Here's the drawing with two shaded views (mm, measured from the low corner). I have some questions. A direction names the side the tool comes from. Give positions to 0.01 mm unless a question says otherwise; leave off trailing zeros. Write each loop counter-clockwise with the first axis right and the second up, starting at its lowest first coordinate (ties: lowest second). Pieces come first, ordered by that corner, then holes.
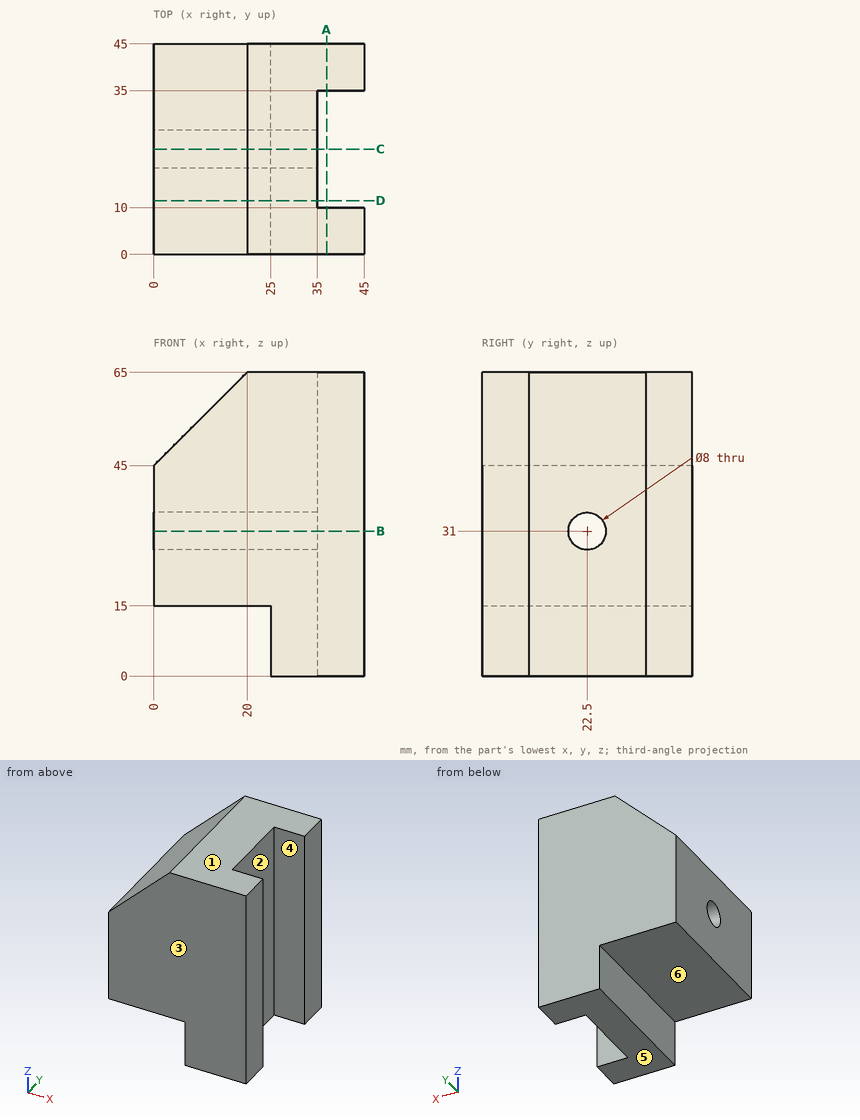
1) Suppose I cut it at A-A on x = 37. Write out the boundary of the cut face in (y, z).
Values follow:
outline: (0, 0) - (10, 0) - (10, 65) - (0, 65) - close; (35, 0) - (45, 0) - (45, 65) - (35, 65) - close
2) Suppose I cut it at B-B on z = 31. Write out the boundary of the cut face in (x, y).
Values follow:
outline: (0, 0) - (45, 0) - (45, 10) - (35, 10) - (35, 18.5) - (0, 18.5) - close; (0, 26.5) - (35, 26.5) - (35, 35) - (45, 35) - (45, 45) - (0, 45) - close
3) If we mould it in two halves opening along Y, with no side actions, what happens to the marked faces 1, 2 and 3? For each: +Y half, -Y half, draft (parallel to the pull), parting line (faces both ways), or undercut.
Values follow:
face 1: draft
face 2: undercut
face 3: -Y half
4) Suppose I cut it at C-C on y = 22.5. Write out the boundary of the cut face in (x, z).
Values follow:
outline: (0, 15) - (25, 15) - (25, 0) - (35, 0) - (35, 27) - (0, 27) - close; (0, 35) - (35, 35) - (35, 65) - (20, 65) - (0, 45) - close
5) Suppose I cut it at D-D on y = 11.5. Write out the boundary of the cut face in (x, z), plus the area to 3 significant figures.
Values follow:
outline: (0, 15) - (25, 15) - (25, 0) - (35, 0) - (35, 65) - (20, 65) - (0, 45) - close
area: 1,700 mm2
6) For pin 1 Ø2 at (x, y) = (17, 22.5) entering from -Z; pin 2 Ø7.5 at (y, z) = (11.5, 9) entering from -X; pin 3 Ø2 at (x, y) = (9.5, 6) entering from +Z, each with a flat end and sliding along its axis, tell me the tip position at first contact or that it passes through.
Values follow:
pin 1: stops at z = 15
pin 2: stops at x = 25
pin 3: stops at z = 55.5
7) For the marked faces 4, 5 and 6, which set-ups out of +Z, -Z, +X, -X, +Y, -Y let a thin tool reach every point of the face, with its end or its side?
Values follow:
face 4: +Z, -Z, +X
face 5: -Z, +X, -X, +Y, -Y
face 6: -Z, -X, +Y, -Y
8) Please list where these lines run through material, in increasing order: L1, parallel to Z at x = 21, y = 22.5; L2, parallel to Y at x = 37, z = 33; L3, parallel to X at y = 14, z = 27.5.
Values follow:
L1: z = 15 to 27, 35 to 65
L2: y = 0 to 10, 35 to 45
L3: x = 0 to 35
